Check sheet for the modelled part. Datum: model origin and axes. Units: mm. Face numbers are marked on the shaded views. A direction names the side the tool comes from. Round coordinates to 2 decimals unless told otherwise and drop trailing zeros. Write each loop counter-clockwise with the first axis right and the second up, starting at its lowest first coordinate (ties: lowest second). Pieces come first, ordered by that corner, then holes. Notation, with made-up numbers: M 25,2 L 71,2 A11 ccw 71,16 Z; hole C 18,86 d2. An arc over 180 degrees is marked long. Answer in a Markdown table with one row per item.
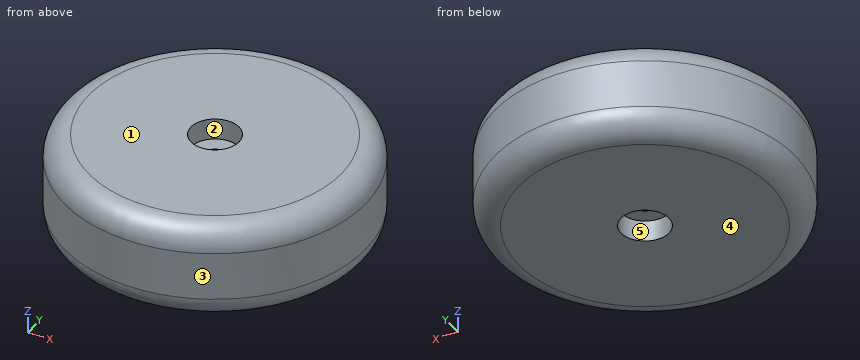
```python
from build123d import *

# Parameters (mm, degrees)
SKETCH_1_R          = 50
EXTRUDE_1_DEPTH     = 32
SKETCH_2_R          = 2.75
CUT_EXTRUDE_1_DEPTH = 78.614431648
FILLET_1_R          = 8
SKETCH_3_R          = 8
CUT_EXTRUDE_2_DEPTH = 7
CUT_EXTRUDE_START   = -7
SKETCH_4_R          = 8
CUT_EXTRUDE_3_DEPTH = 7


with BuildPart() as part:
    # 草图1 → 凸台-拉伸1 (new body)
    with BuildSketch(Plane.XY):
        Circle(SKETCH_1_R)
    extrude(amount=EXTRUDE_1_DEPTH)

    # 草图2 → 切除-拉伸1 (cut, through all)
    with BuildSketch(Plane.XY.offset(32)):
        Circle(SKETCH_2_R)
    extrude(amount=-CUT_EXTRUDE_1_DEPTH, mode=Mode.SUBTRACT)

    # 圆角1
    fillet_1_edges = [part.edges().sort_by_distance(p)[0] for p in [
        (-50, 0, 0),
        (-50, 0, 32),
    ]]
    fillet(fillet_1_edges, radius=FILLET_1_R)

    # 草图3 → 切除-拉伸2 (cut)
    with BuildSketch(Plane.XY.offset(32)):
        Circle(SKETCH_3_R)
    extrude(amount=-CUT_EXTRUDE_2_DEPTH, mode=Mode.SUBTRACT)

    # 草图4 → 切除-拉伸3 (cut)
    with BuildSketch(Plane(origin=(0, 0, 0), x_dir=(-1, 0, 0), z_dir=(0, 0, -1)).offset(CUT_EXTRUDE_START)):
        with Locations(Location((0, 0, 0), (0, 0, 180))):
            Circle(SKETCH_4_R)
    extrude(amount=CUT_EXTRUDE_3_DEPTH, mode=Mode.SUBTRACT)


solid = part.part
```
1. Access from +Z, -Z, +X, -X, +Y, -Y to the whole of each face (thin tool, end or side, straight path). Record for the marked faces 4 and 5.
Found:
| item | result |
|---|---|
| face 4 | -Z, +X, -X, +Y, -Y |
| face 5 | -Z |
2. Section check C-C, the plane z = 5. Record the cut outline in (x, y), and give its area (3 significant figures).
Found:
| item | result |
|---|---|
| outline | C 0,0 d98.83; hole C 0,0 d16 |
| area | 7,470 mm2 |
3. Scan lines: L1, parallel to Y at x = 0, z = 11; L2, parallel to Y at x = 0, z = 30.25; L3, parallel to X at y = -20, z = 2. Record each from-to range of solid material in increasing order.
Found:
| item | result |
|---|---|
| L1 | y = -50 to -2.75, 2.75 to 50 |
| L2 | y = -46.99 to -8, 8 to 46.99 |
| L3 | x = -42.85 to 42.85 |
4. Section check D-D, the plane z = 13. Record the cut outline in (x, y), and give its area (3 significant figures).
Found:
| item | result |
|---|---|
| outline | C 0,0 d100; hole C 0,0 d5.5 |
| area | 7,830 mm2 |
5. Go/stop test with flat-tipped pins: pin 1 (2 mm diameter, centred on y = -8, z = 27, fed in from +X); pin 2 (1 mm diameter, centred on x = -17, z = 25, fed in from -Y); pin 3 (10 mm diameter, centred on x = 3.5, z = 12.5, fed in from +Y); pin 4 (17.5 mm diameter, centred on x = -4, y = -3, fed in from -Z). Record where each tip stops, or that it passes through.
Found:
| item | result |
|---|---|
| pin 1 | stops at x = 49.14 |
| pin 2 | stops at y = -47.14 |
| pin 3 | stops at y = 50 |
| pin 4 | stops at z = 0 |
6. Draft check along Y on the marked faces 1, 2 and 3. Enter one of: +Y half, -Y half, draft (parallel to the pull), parting line (faces both ways), or undercut.
Found:
| item | result |
|---|---|
| face 1 | draft |
| face 2 | undercut |
| face 3 | parting line |
7. Section check A-A, the plane y = 0. Record the cut outline in (x, z), and give its area (3 significant figures).
Found:
| item | result |
|---|---|
| outline | M -50,8 A8 ccw -42,0 L -8,0 L -8,7 L -2.75,7 L -2.75,25 L -8,25 L -8,32 L -42,32 A8 ccw -50,24 Z; M 2.75,7 L 8,7 L 8,0 L 42,0 A8 ccw 50,8 L 50,24 A8 ccw 42,32 L 8,32 L 8,25 L 2.75,25 Z |
| area | 2,820 mm2 |
